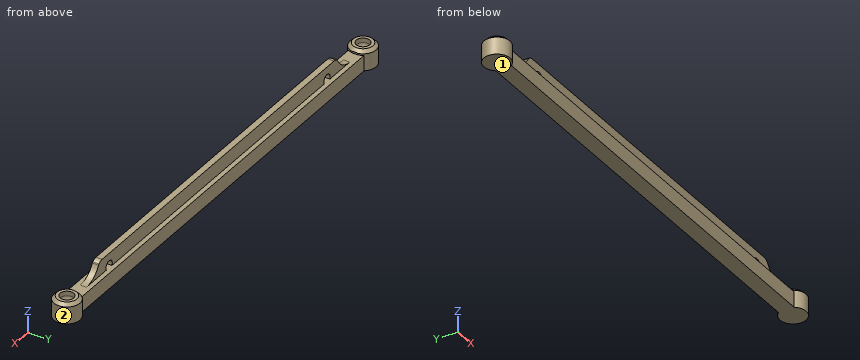
```python
from build123d import *

# Parameters (mm, degrees)
EXTRUDE_1_REACH                  = 81.748
EXTRUDE_1_END_RADIUS             = 4.2
EXTRUDE_1_DIRECTION_2_REACH      = 81.748
EXTRUDE_1_DIRECTION_2_END_RADIUS = 4.2
CUT_EXTRUDE_2_DEPTH              = 155.592270182
CUT_EXTRUDE_3_DEPTH              = 155.592270182


with BuildPart() as part:
    # Sketch 1 → Revolve 2 (revolve)
    with BuildSketch(Plane(origin=(0, 0, 0), x_dir=(0, 0, -1), z_dir=(1, 0, 0))):
        with BuildLine():
            Line((-6.500191237, 4.698061575), (-5.000191237, 4.698061575))
            ThreePointArc((-5.000191237, 4.698061575), (-3.517605127, 4.040424575), (-3.010022497, 2.5))
            Line((-3.010022497, 2.5), (0, 2.5))
            Line((0, 2.5), (0, 6.7))
            Line((0, 6.7), (-5.5, 6.7))
            Line((-5.5, 6.7), (-6.500191237, 5.698061575))
            Line((-6.500191237, 5.698061575), (-6.500191237, 4.698061575))
        make_face()
    revolve(axis=Axis((0, 2.5, -8.961352657), (0, 0, 1)))



with BuildPart() as body_2:
    # Sketch 2 → Revolve 3 (revolve)
    with BuildSketch(Plane(origin=(150, 0, 0), x_dir=(0, 0, -1), z_dir=(1, 0, 0)), mode=Mode.PRIVATE) as revolve_3_sk:
        with BuildLine():
            Line((0, 2.5), (0, 6.7))
            Line((0, 6.7), (-5.5, 6.7))
            Line((-5.5, 6.7), (-6.500191237, 5.698061575))
            Line((-6.500191237, 5.698061575), (-6.500191237, 4.698061575))
            Line((-6.500191237, 4.698061575), (-5.000191237, 4.698061575))
            ThreePointArc((-5.000191237, 4.698061575), (-3.517605127, 4.040424575), (-3.010022497, 2.5))
            Line((-3.010022497, 2.5), (0, 2.5))
        make_face()
    revolve(revolve_3_sk.sketch.rotate(Axis((150, 2.5, 3.010022497), (0, 0, -1)), 180), axis=Axis((150, 2.5, 3.010022497), (0, 0, -1)))


with BuildPart() as part_1:
    add(part.part)

    add(body_2.part)  # Extrude 1 merges body 2
    # Extrude 1: up to this cylinder (the profile starts outside it)
    extrude_1_end = Plane(origin=(150, 2.5, 3.825291), z_dir=(0, 0, 1)) * Cylinder(EXTRUDE_1_END_RADIUS, 172.896, mode=Mode.PRIVATE)
    # Sketch 3 → Extrude 1 (add, up to the surface)
    with BuildSketch(Plane(origin=(75, 0, 0), x_dir=(0, 0, -1), z_dir=(1, 0, 0)), mode=Mode.PRIVATE) as extrude_1_sk1:
        Polygon((-5, 3.5), (-5, 5), (0, 5), (0, 0), (-5, 0), (-5, 1.5), (-9.7, 1.5), (-9.7, 3.5), align=None)
    extrude_1_tool1 = extrude(extrude_1_sk1.sketch, amount=EXTRUDE_1_REACH, mode=Mode.PRIVATE) - extrude_1_end
    add(extrude_1_tool1.solids().sort_by_distance((75, 2.5, 3.825291))[0])

    # Extrude 1 direction 2: up to this cylinder (the profile starts outside it)
    extrude_1_direction_2_end = Plane(origin=(0, 2.5, 3.825291), z_dir=(0, 0, -1)) * Cylinder(EXTRUDE_1_DIRECTION_2_END_RADIUS, 172.896, mode=Mode.PRIVATE)
    # Sketch 3 → Extrude 1 direction 2 (add, up to the surface)
    with BuildSketch(Plane(origin=(75, 0, 0), x_dir=(0, 0, -1), z_dir=(1, 0, 0)), mode=Mode.PRIVATE) as extrude_1_direction_2_sk1:
        Polygon((-5, 3.5), (-5, 5), (0, 5), (0, 0), (-5, 0), (-5, 1.5), (-9.7, 1.5), (-9.7, 3.5), align=None)
    extrude_1_direction_2_tool1 = extrude(extrude_1_direction_2_sk1.sketch, amount=-EXTRUDE_1_DIRECTION_2_REACH, mode=Mode.PRIVATE) - extrude_1_direction_2_end
    add(extrude_1_direction_2_tool1.solids().sort_by_distance((75, 2.5, 3.825291))[0])

    # Sketch 4 → Cut-Extrude 2 (cut, through all)
    with BuildSketch(Plane.XZ.offset(-1.5)):
        with BuildLine():
            Line((145.920784389, 9.7), (133.73, 9.7))
            ThreePointArc((133.73, 9.7), (134.59, 9.536801651), (135.330428215, 9.069897208))
            Line((135.330428215, 9.069897208), (135.567873872, 8.812759968))
            ThreePointArc((135.567873872, 8.812759968), (138.083605002, 6.031129475), (141.689592152, 5))
            Line((141.689592152, 5), (145.920784389, 5))
            Line((145.920784389, 5), (145.920784389, 9.7))
        make_face()
        with BuildLine():
            ThreePointArc((14.669571785, 9.069897208), (15.41, 9.536801651), (16.27, 9.7))
            Line((16.27, 9.7), (4.079215611, 9.7))
            Line((4.079215611, 9.7), (4.079215611, 5))
            Line((4.079215611, 5), (8.310407839, 5))
            ThreePointArc((8.310407839, 5), (11.916394994, 6.031129473), (14.432126128, 8.812759968))
            Line((14.432126128, 8.812759968), (14.669571785, 9.069897208))
        make_face()
    extrude(amount=-CUT_EXTRUDE_2_DEPTH, mode=Mode.SUBTRACT)

    # Sketch 6 → Cut-Extrude 3 (cut, through all)
    with BuildSketch(Plane.XZ.offset(-1.5)):
        with BuildLine():
            ThreePointArc((21.233, 5), (19.7945, 7.300512491), (18.356, 5))
            Line((18.356, 5), (21.233, 5))
        make_face()
        with BuildLine():
            ThreePointArc((131.644, 5), (130.2055, 7.300512491), (128.767, 5))
            Line((128.767, 5), (131.644, 5))
        make_face()
    extrude(amount=-CUT_EXTRUDE_3_DEPTH, mode=Mode.SUBTRACT)


solid = part_1.part
```
Model file for the job. Use its own axes, mm. Face numbers are marked on the shaded views. Round coordinates to 2 decimals unless told otherwise and drop trailing zeros. Order: outer loops, then holes, each group sorted by start corner. A loop starts at its lowest first (then second) coordinate and runs counter-clockwise, first axis right, second up. Notation, with made-up numbers: M 67.5,22 L 75.5,22 A21 ccw 75.5,46 Z; hole C -24.5,8.25 d5. An arc over 180 degrees is marked long. Use CSV: the item, a comma, the result in double quotes.
Item 1: Saw through at A-A (x = 48). List the corners of the cut face in (y, z), plus the area to 3 significant figures.
Worked answers:
outline,"M 0,0 L 5,0 L 5,5 L 3.5,5 L 3.5,9.7 L 1.5,9.7 L 1.5,5 L 0,5 Z"
area,"34.4 mm²"
Item 2: Saw through at B-B (x = 7). List the corners of the cut face in (y, z).
Worked answers:
outline,"M 0,0 L 5,0 L 5,5 L 0,5 Z"
Item 3: Pin check, flat tips, straight feed: pin 1 (4 mm diameter, centred on x = 130.21, z = 5.7, fed in from +Y); pin 2 (1.4 mm diameter, centred on x = 91, z = 7.5, fed in from -Y); pin 3 (5.5 mm diameter, centred on x = 97.5, z = 2.5, fed in from -Y). Stop position of each tip, or through.
Worked answers:
pin 1,"y = 5"
pin 2,"y = 1.5"
pin 3,"y = 0"
Item 4: Probe probe 1 along X at (y, z) = (4, 4); probe 2 along Z at (x, y) = (109.5, 0.5); probe 3 along X at (y, z) = (3, 2.5). List the from-to ranges inside material, lowest first.
Worked answers:
probe 1,"-3.92 to -1.21, 1.21 to 148.79, 151.21 to 153.92"
probe 2,"0 to 5"
probe 3,"-4.17 to 154.17"
Item 5: Pull direction X, two halves, no side cores. Call the marked faces 1 and 2: released by +X, released by -X, zero draft, split by the parting line, or undercut.
Worked answers:
face 1,"zero draft"
face 2,"undercut"
